```python
from build123d import *

# Parameters (mm, degrees)
SKETCH1_W           = 22.0472
SKETCH1_H           = 30.0736
BOSS_EXTRUDE1_DEPTH = 28.194
SKETCH2_R           = 1.5875
CUT_EXTRUDE1_DEPTH  = 4.826
SKETCH3_R           = 5.7531
CUT_EXTRUDE2_DEPTH  = 13.462
SKETCH4_R           = 5.7531
CUT_EXTRUDE3_DEPTH  = 13.462
FILLET1_R           = 0.762


with BuildPart() as part:
    # Sketch1 → Boss-Extrude1 (new body)
    with BuildSketch(Plane(origin=(0, 0, 0), x_dir=(1, 0, 0), z_dir=(0, 1, 0))):
        with Locations((11.0236, 15.0368)):
            Rectangle(SKETCH1_W, SKETCH1_H)
    extrude(amount=BOSS_EXTRUDE1_DEPTH)

    # Sketch2 → Cut-Extrude1 (cut)
    with BuildSketch(Plane.XZ):
        with Locations((3.2131, -5.2705)):
            Circle(SKETCH2_R)
        with Locations((18.7071, -5.2705)):
            Circle(SKETCH2_R)
    extrude(amount=-CUT_EXTRUDE1_DEPTH, mode=Mode.SUBTRACT)

    # Sketch3 → Cut-Extrude2 (cut)
    with BuildSketch(Plane.XY):
        with Locations((11.1379, 9.9441)):
            Circle(SKETCH3_R)
    extrude(amount=-CUT_EXTRUDE2_DEPTH, mode=Mode.SUBTRACT)

    # Sketch4 → Cut-Extrude3 (cut)
    with BuildSketch(Plane(origin=(0, 0, -30.0736), x_dir=(-1, 0, 0), z_dir=(0, 0, -1))):
        with Locations((-10.9093, 9.7917)):
            Circle(SKETCH4_R)
    extrude(amount=-CUT_EXTRUDE3_DEPTH, mode=Mode.SUBTRACT)

    # Fillet1
    fillet1_edges = [part.edges().sort_by_distance(p)[0] for p in [
        (0, 14.097, -30.0736),
        (22.0472, 14.097, -30.0736),
        (22.0472, 14.097, 0),
        (0, 14.097, 0),
    ]]
    fillet(fillet1_edges, radius=FILLET1_R)


solid = part.part
```
The listing builds one solid part. Answer for the finished solid, in the listing's coordinates (mm). A direction names the side the tool comes from. Give positions to 0.01 mm unless a question says otherwise; leave off trailing zeros. Loops run counter-clockwise (first coordinate to the right, second up) from the corner with the lowest first, then second, coordinate; pieces in that order, holes last. Notation, with made-up numbers: M 26.5,38.5 L 70.5,38.5 A8 cw 70.5,43.5 Z; hole C 60,-14 d7. An arc over 180 degrees is marked long. One line per item, written item: value.
Q1. Flat-ended cylindrical pins translate along their axes: P1, Ø12.5, axis at x = 8, y = 8.5, coming from the -Z side; P2, Ø1.5, axis at x = 10, y = 13, coming from the +Z side; P3, Ø1, axis at x = 3.5, z = -5.5, coming from the -Y side. Find the tip coordinate at first contact, or state that the pin passes through.
Working result:
P1: stops at z = -30.07
P2: stops at z = -13.46
P3: stops at y = 4.83
Q2. A cutting plane is placed at A-A on y = 3.25. Determine the outline of the cut face in (x, z) (1 decimal).
Working result:
outline: M 0,-29.3 A0.8 ccw 0.8,-30.1 L 21.3,-30.1 A0.8 ccw 22,-29.3 L 22,-0.8 A0.8 ccw 21.3,0 L 0.8,0 A0.8 ccw 0,-0.8 Z; hole C 3.2,-5.3 d3.2; hole C 18.7,-5.3 d3.2
Q3. For faces 1 (the face through (11, 17, 0)), 2 (the face through (11, 10, -13.462)), 3 (the face through (3.006, 2.379, -3.697)), 4 (the face through (11, 10, -16.612)), 5 (the face through (22.047, 14, -15)), determine the directions among +Z, -Z, +X, -X, +Y, -Y from which every point of the face is accessible in a straight line to the end or side of a thin tool.
Working result:
face 1: +Z, +X, -X, +Y, -Y
face 2: +Z
face 3: -Y
face 4: -Z
face 5: +Z, -Z, +X, +Y, -Y
Q4. A cutting plane is placed at B-B on x = 13. Determine the outline of the cut face in (y, z), then the cut area to 3 significant figures.
Working result:
outline: M 0,-30.07 L 4.43,-30.07 L 4.43,-16.61 L 15.15,-16.61 L 15.15,-30.07 L 28.19,-30.07 L 28.19,0 L 15.39,0 L 15.39,-13.46 L 4.5,-13.46 L 4.5,0 L 0,0 Z
area: 557 mm^2
Q5. Find the intervals of material crossed by line 1 (Z direction, x = 12.5, y = 13); line 2 (X direction, y = 6.75, z = -6); line 3 (X direction, y = 8, z = -25), in increasing order. Write a range as from..to.
Working result:
line 1: z = -16.61..-13.46
line 2: x = 0..6.35, 15.92..22.05
line 3: x = 0..5.44, 16.38..22.05
Q6. A cutting plane is placed at D-D on y = 6.25. Determine the outline of the cut face in (x, z).
Working result:
outline: M 0,-29.31 A0.76 ccw 0.76,-30.07 L 6.38,-30.07 L 6.38,-16.61 L 15.44,-16.61 L 15.44,-30.07 L 21.29,-30.07 A0.76 ccw 22.05,-29.31 L 22.05,-0.76 A0.76 ccw 21.29,0 L 15.55,0 L 15.55,-13.46 L 6.73,-13.46 L 6.73,0 L 0.76,0 A0.76 ccw 0,-0.76 Z
Q7. A cutting plane is placed at C-C on z = -13. Determine the outline of the cut face in (x, y).
Working result:
outline: M 0,0 L 22.05,0 L 22.05,28.19 L 0,28.19 Z; hole C 11.14,9.94 d11.51
Q8. Determine the mould class of faces 6 (the face through (19, 4.826, -5)), 7 (the face through (11, 28.194, -15)), 8 (the face through (0, 14, -15)) for opening direction X: +X half, -X half, draft (parallel to the pull), parting line (faces both ways), or undercut.
Working result:
face 6: undercut
face 7: draft
face 8: -X half
